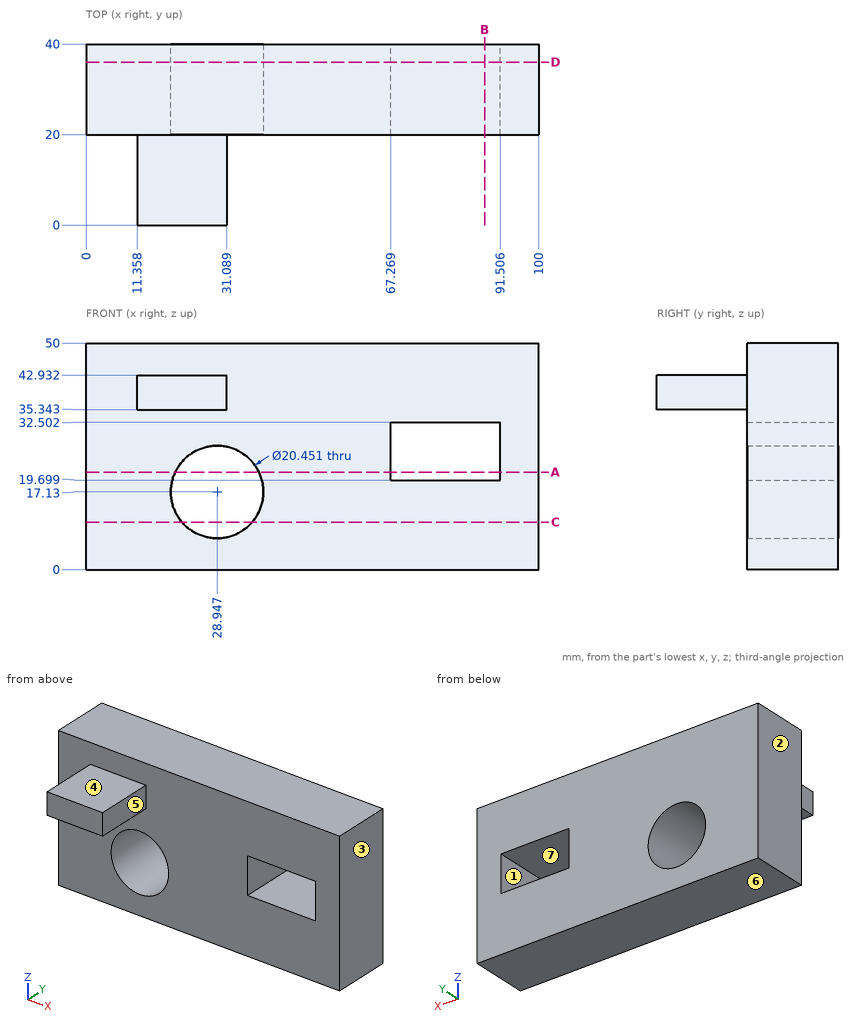
Study the drawing (mm; zero at the part's minimum x, y, z) and answer. A direction names the side the tool comes from. Coordinates: 2 decimals unless noted, no trailing zeros. Loops run counter-clockwise (first coordinate to the right, second up) from the corner with the lowest first, then second, coordinate; pieces in that order, holes last. Notation, with made-up numbers: (11, -15.5) -> (35, -15.5) arc R17 cw to (35, -2.5) -> close; hole circle Ø6 at (15.5, 23.5). An arc over 180 degrees is marked (long way). Write item = value, one per line. Start each with the question number.
1) The mould has two halves that part along X. Classify the marked faces 1, 2 and 3: pulls with the +X half, pulls with the -X half, needs draft (parallel to the pull), parting line crosses it, or undercut.
2) Given P1, Ø6, axis at x = 19, y = 6.5, coming from the +Z side; P2, Ø25, axis at x = 26.5, z = 21.5, coming from the -Y side; P3, Ø2.5, axis at y = 13.5, z = 40, coming from the +X side, each flat-ended and moving along its own axis, determine where each tip first touches the part or whether it passes through.
3) The part is cut by section D-D, the plane y = 36. State how many separate pieces and enclosed holes the cut face has, plus the area to 3 significant figures.
4) For the marked faces 4, 5, 6 and 7, determine the directions among +Z, -Z, +X, -X, +Y, -Y from which every point of the face is accessible in a straight line to the end or side of a thin tool.
5) The part is cut by section C-C, the plane z = 10.5. Determine the outline of the cut face in (x, y), plus the area to 3 significant figures.
6) Find the intervals of material crossed by L1, parallel to Z at x = 75, y = 36; L2, parallel to Y at x = 46, z = 26.5; L3, parallel to Z at x = 37, y = 22 (1 decimal), in increasing order. Write a range as from..to.
7) The part is cut by section B-B, the plane x = 88. Determine the outline of the cut face in (y, z).
8) The part is cut by section A-A, the plane z = 21.5. Determine the outline of the cut face in (x, y).
Result:
q1.face_1 = undercut
q1.face_2 = pulls with the -X half
q1.face_3 = pulls with the +X half
q2.P1 = 42.93
q2.P2 = 20
q2.P3 = 31.09
q3.separate_pieces = 1
q3.enclosed_holes = 2
q3.area = 4,360 mm²
q4.face_4 = +Z, +X, -X, -Y
q4.face_5 = +Z, -Z, +X, -Y
q4.face_6 = -Z, +X, -X, +Y, -Y
q4.face_7 = +Y, -Y
q5.outline = (0, 20) -> (21.16, 20) -> (21.16, 40) -> (0, 40) -> close; (36.73, 20) -> (100, 20) -> (100, 40) -> (36.73, 40) -> close
q5.area = 1,690 mm²
q6.L1 = 0..19.7, 32.5..50
q6.L2 = 20..40
q6.L3 = 0..10.8, 23.4..50
q7.outline = (20, 0) -> (40, 0) -> (40, 19.7) -> (20, 19.7) -> close; (20, 32.5) -> (40, 32.5) -> (40, 50) -> (20, 50) -> close
q8.outline = (0, 20) -> (19.7, 20) -> (19.7, 40) -> (0, 40) -> close; (38.19, 20) -> (67.27, 20) -> (67.27, 40) -> (38.19, 40) -> close; (91.51, 20) -> (100, 20) -> (100, 40) -> (91.51, 40) -> close
